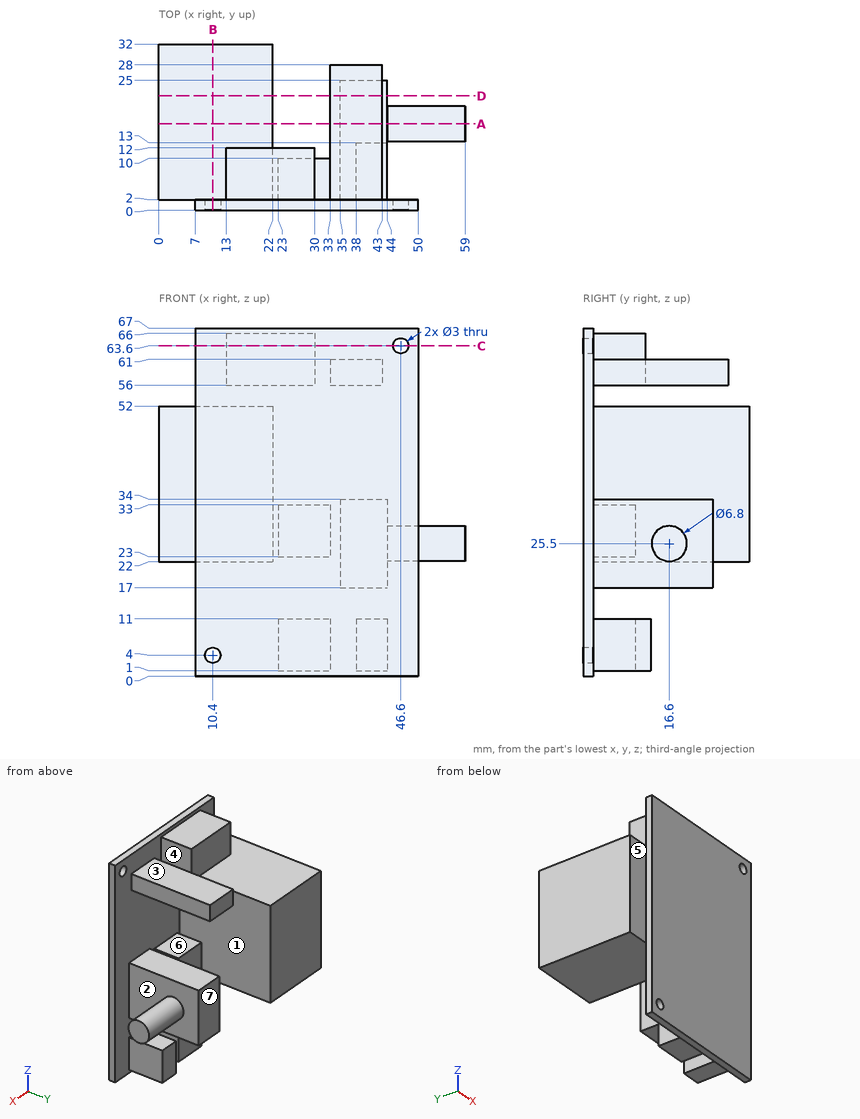
Drawing for the job (mm, zero at the part's lowest x, y, z). A direction names the side the tool comes from. Give positions to 0.01 mm unless a question says otherwise; leave off trailing zeros. Loops run counter-clockwise (first coordinate to the right, second up) from the corner with the lowest first, then second, coordinate; pieces in that order, holes last. Notation, with made-up numbers: M -34,30.25 L -18,30.25 A24 ccw -18,44.25 Z; hole C 5.25,12.25 d6. An arc over 180 degrees is marked long. One line per question, with ' | ' between items. Start each with the question number.
1. Saw through at C-C on z = 63.6. Give the cut face in (x, y).
2. Saw through at D-D on y = 22. Give the cut face in (x, z), plus the area to 3 significant figures.
3. Two-plate mould, pull along X, no slides. Class the marked faces 1, 2, 3 and 4: pulls with the +X half, pulls with the -X half, needs draft (parallel to the pull), parting line crosses it, or undercut.
4. Flat gauge pins, fed straight in: pin 1 (2.5 mm diameter, centred on x = 40.5, z = 28, fed in from +Y); pin 2 (1 mm diameter, centred on y = 15, z = 59, fed in from +X); pin 3 (2 mm diameter, centred on x = 30, z = 51.5, fed in from +Y). Where does each tip first touch, or does it go through?
5. 3-axis set-ups, long thin cutter, end or side, ignore diameter. For the marked faces 5, 6 and 7: which of +Z, -Z, +X, -X, +Y, -Y reach the whole face in a straight line?
6. Saw through at A-A on y = 16.6. Give the cut face in (x, z), plus the area to 3 significant figures.
7. Saw through at B-B on x = 10.4. Give the cut face in (y, z).
8. Probe L1, parallel to X at y = 9, z = 25; L2, parallel to Z at x = 39.5, y = 12; L3, parallel to X at y = 1.4, z = 4. List the from-to ranges inside material, lowest first. Write a range as from..to.
Result sheet:
1) outline: M 7,0 L 45.1,0 L 45.1,2 L 30,2 L 30,12 L 13,12 L 13,2 L 7,2 Z; M 48.1,0 L 50,0 L 50,2 L 48.1,2 Z
2) outline: M 0,22 L 22,22 L 22,52 L 0,52 Z; M 33,56 L 43,56 L 43,61 L 33,61 Z; M 35,17 L 44,17 L 44,34 L 35,34 Z | area: 863 mm^2
3) face 1: undercut | face 2: pulls with the +X half | face 3: needs draft | face 4: undercut
4) pin 1: stops at y = 25 | pin 2: stops at x = 43 | pin 3: stops at y = 2
5) face 5: +Z, -Z, -X, -Y | face 6: +Y | face 7: -Z, +X, +Y
6) outline: M 0,22 L 22,22 L 22,52 L 0,52 Z; M 33,56 L 43,56 L 43,61 L 33,61 Z; M 35,17 L 44,17 L 44,22.1 L 59,22.1 L 59,28.9 L 44,28.9 L 44,34 L 35,34 Z | area: 965 mm^2
7) outline: M 0,0 L 2,0 L 2,2.5 L 0,2.5 Z; M 0,5.5 L 2,5.5 L 2,22 L 32,22 L 32,52 L 2,52 L 2,67 L 0,67 Z
8) L1: x = 0..22, 23..33, 35..44 | L2: z = 1..11, 17..34, 56..61 | L3: x = 7..8.9, 11.9..50
